Build history of the part. All positions in model axes, mm. A direction names the side the tool comes from. Give positions to 0.01 mm unless a question says otherwise; leave off trailing zeros. Loops run counter-clockwise (first coordinate to the right, second up) from the corner with the lowest first, then second, coordinate; pieces in that order, holes last. Notation, with made-up numbers: (7.25, 76.25) -> (55.25, 76.25) arc R38 ccw to (55.25, 115.25) -> close; hole circle Ø4 at (-9.75, 51). An arc over 180 degrees is marked (long way). Answer as a JSON object with one key per item and string values. Group by question number.
Q1. Two-plate mould, pull along Y, no slides. Class faces 1 (the cylindrical face through (0.829, -1.972, -35.936)), 2 (the flat face through (0, -4, -18)), 3 (the flat face through (0, 40, 2)), 4 (the cylindrical face through (-11.323, 15.544, 1.972)): pulls with the +Y half, pulls with the -Y half, needs draft (parallel to the pull), parting line crosses it, or undercut.
Q2. Band-saw the part on A-A, the plane x = 17.5. Write the cut outline in (y, z).
Q3. Band-saw the part on B-B, the plane y = 2.5. Write the cut outline in (x, z), plus the area to 3 significant figures.
Q4. Drop flat-ended pins along their axis: pin 1 (3 mm diameter, centred on x = 8.42, y = 33.56, fed in from +Z); pin 2 (5 mm diameter, centred on x = -1.58, y = 33.56, fed in from -Z); pin 3 (12 mm diameter, centred on x = -1.5, z = -25.5, fed in from +Y). Give the stop position or say it passes through.
Q5. Tool access for faces 5 (the cylindrical face through (16.569, 32.795, 1.972)), 6 (the flat face through (0, 20, 0)): list every direction of +Z, -Z, +X, -X, +Y, -Y with a clear straight run to the whole face (end or side of a thin tool).
Q6. Wall check: probe 1 along Z at (x, y) = (10, -1); probe 2 along Z at (x, y) = (12, 18.5); probe 3 along Y at (x, z) = (20, -8). Give the ranges that are in metal, low to high. Write a range as from..to.
Q7. Band-saw the part on C-C, the plane z = -4.5. Write the cut outline in (x, y).
from build123d import *

# Parameters (mm, degrees)
EXTRUDE_THIN1_DEPTH = 25
SKETCH2_R           = 2
CUT_EXTRUDE1_DEPTH  = 5
SKETCH3_R           = 2
CUT_EXTRUDE2_DEPTH  = 5


with BuildPart() as part:
    # Sketch1 → Extrude-Thin1 (new body, symmetric)
    with BuildSketch(Plane(origin=(0, 0, 0), x_dir=(0, 0, -1), z_dir=(1, 0, 0))):
        Polygon((0, 40), (0, 0), (40, 0), (40, -4), (-4, -4), (-4, 40), align=None)
    extrude(amount=EXTRUDE_THIN1_DEPTH, both=True)

    # Sketch2 → Cut-Extrude1 (cut, through all)
    with BuildSketch(Plane(origin=(0, 0, 0), x_dir=(1, 0, 0), z_dir=(0, 1, 0))):
        with Locations((-18.910875839, 33.953285117)):
            Circle(SKETCH2_R)
        with Locations((-8.910875839, 33.953285117)):
            Circle(SKETCH2_R)
        with Locations((1.089124161, 33.953285117)):
            Circle(SKETCH2_R)
        with Locations((11.089124161, 33.953285117)):
            Circle(SKETCH2_R)
        with Locations((21.089124161, 33.953285117)):
            Circle(SKETCH2_R)
        with Locations((-8.910875839, 23.953285117)):
            Circle(SKETCH2_R)
        with Locations((1.089124161, 23.953285117)):
            Circle(SKETCH2_R)
        with Locations((11.089124161, 23.953285117)):
            Circle(SKETCH2_R)
        with Locations((21.089124161, 23.953285117)):
            Circle(SKETCH2_R)
        with Locations((-8.910875839, 13.953285117)):
            Circle(SKETCH2_R)
        with Locations((1.089124161, 13.953285117)):
            Circle(SKETCH2_R)
        with Locations((11.089124161, 13.953285117)):
            Circle(SKETCH2_R)
        with Locations((21.089124161, 13.953285117)):
            Circle(SKETCH2_R)
        with Locations((-18.910875839, 23.953285117)):
            Circle(SKETCH2_R)
        with Locations((-18.910875839, 13.953285117)):
            Circle(SKETCH2_R)
    extrude(amount=-CUT_EXTRUDE1_DEPTH, mode=Mode.SUBTRACT)

    # Sketch3 → Cut-Extrude2 (cut, through all)
    with BuildSketch(Plane(origin=(0, 0, 0), x_dir=(-1, 0, 0), z_dir=(0, 0, -1))):
        with Locations((-18.416248434, 33.561450044)):
            Circle(SKETCH3_R)
        with Locations((-8.416248434, 33.561450044)):
            Circle(SKETCH3_R)
        with Locations((1.583751566, 33.561450044)):
            Circle(SKETCH3_R)
        with Locations((11.583751566, 33.561450044)):
            Circle(SKETCH3_R)
        with Locations((21.583751566, 33.561450044)):
            Circle(SKETCH3_R)
        with Locations((-8.416248434, 23.561450044)):
            Circle(SKETCH3_R)
        with Locations((1.583751566, 23.561450044)):
            Circle(SKETCH3_R)
        with Locations((11.583751566, 23.561450044)):
            Circle(SKETCH3_R)
        with Locations((21.583751566, 23.561450044)):
            Circle(SKETCH3_R)
        with Locations((-8.416248434, 13.561450044)):
            Circle(SKETCH3_R)
        with Locations((1.583751566, 13.561450044)):
            Circle(SKETCH3_R)
        with Locations((11.583751566, 13.561450044)):
            Circle(SKETCH3_R)
        with Locations((21.583751566, 13.561450044)):
            Circle(SKETCH3_R)
        with Locations((-18.416248434, 23.561450044)):
            Circle(SKETCH3_R)
        with Locations((-18.416248434, 13.561450044)):
            Circle(SKETCH3_R)
    extrude(amount=-CUT_EXTRUDE2_DEPTH, mode=Mode.SUBTRACT)


solid = part.part
Worked answers:
{
 "1": {"face 1": "needs draft", "face 2": "pulls with the -Y half", "face 3": "pulls with the +Y half", "face 4": "undercut"},
 "2": {"outline": "(-4, -40) -> (0, -40) -> (0, 0) -> (11.78, 0) -> (11.78, 4) -> (-4, 4) -> close; (15.34, 0) -> (21.78, 0) -> (21.78, 4) -> (15.34, 4) -> close; (25.34, 0) -> (31.78, 0) -> (31.78, 4) -> (25.34, 4) -> close; (35.34, 0) -> (40, 0) -> (40, 4) -> (35.34, 4) -> close"},
 "3": {"outline": "(-25, 0) -> (25, 0) -> (25, 4) -> (-25, 4) -> close", "area": "200 mm2"},
 "4": {"pin 1": "through", "pin 2": "z = 0", "pin 3": "y = 0"},
 "5": {"face 5": "+Z, -Z", "face 6": "-Z, +X, -X, +Y"},
 "6": {"probe 1": "-40..-35.63, -32.28..-25.63, -22.28..-15.63, -12.28..4", "probe 2": "0..4", "probe 3": "-4..0"},
 "7": {"outline": "(-25, -4) -> (25, -4) -> (25, 0) -> (-25, 0) -> close"}
}
